Print and shaded views of the part. All mm, measured from the part's lowest x, y and z. A direction names the side the tool comes from. Round coordinates to 2 decimals unless told otherwise and drop trailing zeros. Order: outer loops, then holes, each group sorted by start corner. A loop starts at its lowest first (then second) coordinate and runs counter-clockwise, first axis right, second up. Notation, with made-up numbers: (87, 1.5) - (118, 1.5) arc R12 ccw to (118, 5.5) - close; hole circle Ø3 at (64.25, 21.25). An arc over 180 degrees is marked (long way). Write item = value, one per line. Start each with the question number.
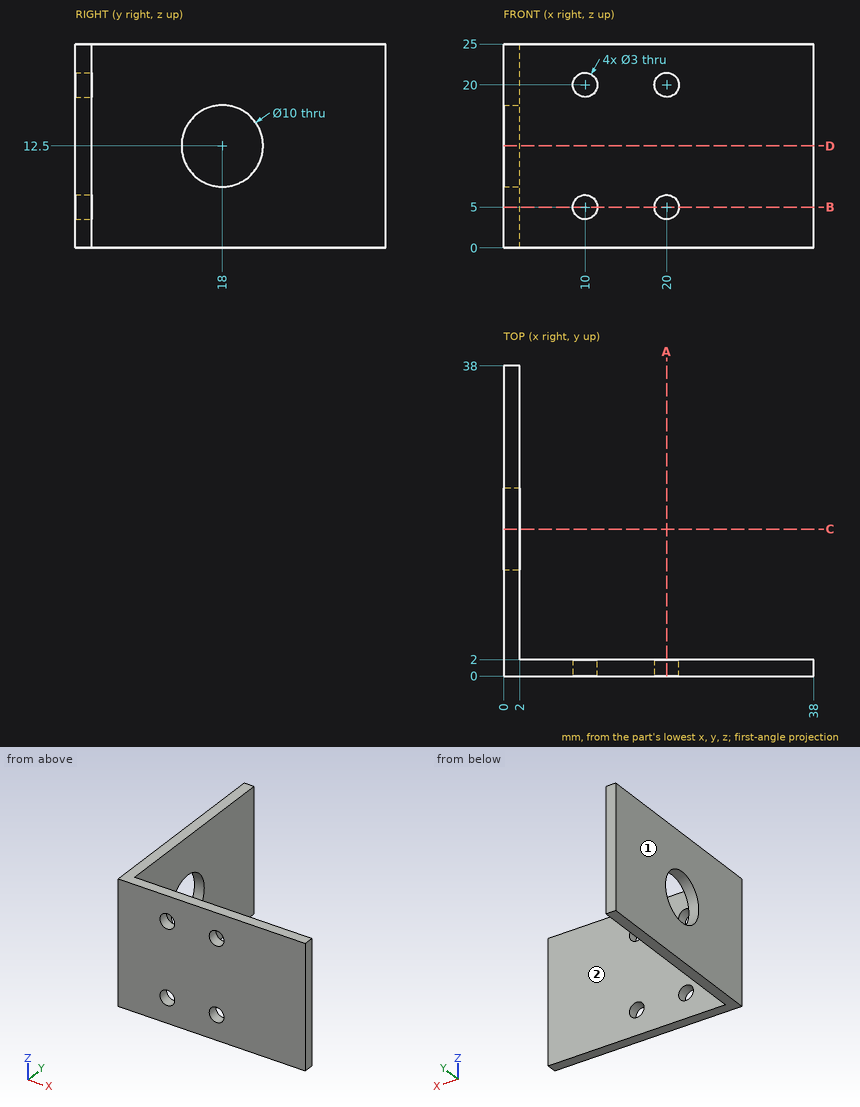
Item 1: Drop flat-ended pins along their axis: pin 1 (8 mm diameter, centred on y = 18, z = 12.5, fed in from +X); pin 2 (12.5 mm diameter, centred on x = 23.5, z = 13.5, fed in from +Y); pin 3 (6 mm diameter, centred on y = 21.5, z = 18.5, fed in from +X). Give the stop position or say it passes through.
Item 2: Saw through at B-B, the plane z = 5. Give the cut face in (x, y), then the cut area to 3 significant figures.
Item 3: Which spindle directions (+Z, -Z, +X, -X, +Y, -Y) get a long thin tool onto all of the face, cutting with end or side? Do the marked faces 1 and 2. Say none if no direction does.
Item 4: Saw through at D-D, the plane z = 12.5. Give the cut face in (x, y).
Item 5: Saw through at C-C, the plane y = 18. Give the cut face in (x, z), then the cut area to 3 significant figures.
Item 6: Saw through at A-A, the plane x = 20. Give the cut face in (y, z).
Item 7: Probe L1, parallel to Z at x = 20, y = 1.1; L2, parallel to X at y = 35, z = 20.75. List the from-to ranges inside material, lowest first.
Check sheet entries:
q1.pin_1 = through
q1.pin_2 = 2
q1.pin_3 = 2
q2.outline = (0, 0) - (8.5, 0) - (8.5, 2) - (2, 2) - (2, 38) - (0, 38) - close; (11.5, 0) - (18.5, 0) - (18.5, 2) - (11.5, 2) - close; (21.5, 0) - (38, 0) - (38, 2) - (21.5, 2) - close
q2.area = 136 mm2
q3.face_1 = +Z, -Z, -X, +Y, -Y
q3.face_2 = +Z, -Z, +X, +Y
q4.outline = (0, 0) - (38, 0) - (38, 2) - (2, 2) - (2, 13) - (0, 13) - close; (0, 23) - (2, 23) - (2, 38) - (0, 38) - close
q5.outline = (0, 0) - (2, 0) - (2, 7.5) - (0, 7.5) - close; (0, 17.5) - (2, 17.5) - (2, 25) - (0, 25) - close
q5.area = 30.0 mm2
q6.outline = (0, 0) - (2, 0) - (2, 3.5) - (0, 3.5) - close; (0, 6.5) - (2, 6.5) - (2, 18.5) - (0, 18.5) - close; (0, 21.5) - (2, 21.5) - (2, 25) - (0, 25) - close
q7.L1 = 0 to 3.5, 6.5 to 18.5, 21.5 to 25
q7.L2 = 0 to 2
